Design review of the part built by this model. Coordinates are the model's own, in mm. A direction names the side the tool comes from. Give positions to 0.01 mm unless a question says otherwise; leave off trailing zeros. Write each loop counter-clockwise with the first axis right and the second up, starting at its lowest first coordinate (ties: lowest second). Pieces come first, ordered by that corner, then holes. Notation, with made-up numbers: (9, -20) -> (44, -20) arc R19 cw to (44, -15) -> close; hole circle Ø5 at (40.5, -22.5). An arc over 180 degrees is marked (long way). Answer as a JSON object with one key per item and string values.
```python
from build123d import *

# Parameters (mm, degrees)
F0_R     = 12.5
F1_DEPTH = 20
F2_R     = 50
F3_DEPTH = 40
F4_R     = 34.837403
F5_DEPTH = 100
F7_DEPTH = 25


with BuildPart() as f1:
    # F0 (on Top) → F1 (new body)
    with BuildSketch(Plane.XY):
        with BuildLine():
            ThreePointArc((100, 80), (94.142136, 94.142136), (80, 100))
            Line((80, 100), (-80, 100))
            ThreePointArc((-80, 100), (-94.142136, 94.142136), (-100, 80))
            Line((-100, 80), (-100, -80))
            ThreePointArc((-100, -80), (-94.142136, -94.142136), (-80, -100))
            Line((-80, -100), (80, -100))
            ThreePointArc((80, -100), (94.142136, -94.142136), (100, -80))
            Line((100, -80), (100, 80))
        make_face()
        with Locations((-77, -77)):
            Circle(F0_R, mode=Mode.SUBTRACT)
        with Locations((77, -77)):
            Circle(F0_R, mode=Mode.SUBTRACT)
        with Locations((-77, 77)):
            Circle(F0_R, mode=Mode.SUBTRACT)
        with Locations((77, 77)):
            Circle(F0_R, mode=Mode.SUBTRACT)
    extrude(amount=-F1_DEPTH)

    # F2 (on face) → F3 (join)
    with BuildSketch(Plane.XY):
        Circle(F2_R)
    extrude(amount=F3_DEPTH)

    # F4 (on face) → F5 (cut)
    with BuildSketch(Plane.XY.offset(40)):
        Circle(F4_R)
    extrude(amount=-F5_DEPTH, mode=Mode.SUBTRACT)

    # F6 (on Top) → F7 (cut)
    with BuildSketch(Plane.XY):
        with BuildLine():
            ThreePointArc((-59.309852, -34.015045), (-68.347947, 1.800006), (-57.437243, 37.089687))
            ThreePointArc((-57.437243, 37.089687), (-62.013533, 48.246062), (-74.069896, 48.019696))
            ThreePointArc((-74.069896, 48.019696), (-88.19022, 3.83743), (-77.961014, -41.40436))
            ThreePointArc((-77.961014, -41.40436), (-77.365723, -42.506301), (-76.754857, -43.599686))
            ThreePointArc((-76.754857, -43.599686), (-63.805315, -46.501), (-59.309852, -34.015045))
        make_face()
        with BuildLine():
            ThreePointArc((-77.961014, -41.40436), (-77.426731, -42.53982), (-76.754857, -43.599686))
            ThreePointArc((-76.754857, -43.599686), (-77.365723, -42.506301), (-77.961014, -41.40436))
        make_face()
        with BuildLine():
            ThreePointArc((-54.052199, 69.789687), (-53.014186, 70.58142), (-51.964577, 71.357714))
            ThreePointArc((-51.964577, 71.357714), (-53.059588, 70.641867), (-54.052199, 69.789687))
        make_face()
        with BuildLine():
            ThreePointArc((52.94881, 70.630476), (0.61188, 88.271549), (-51.964577, 71.357714))
            ThreePointArc((-51.964577, 71.357714), (-53.014186, 70.58142), (-54.052199, 69.789687))
            ThreePointArc((-54.052199, 69.789687), (-55.057173, 56.587711), (-42.098027, 53.874279))
            ThreePointArc((-42.098027, 53.874279), (1.351238, 68.358291), (44.194175, 52.168541))
            ThreePointArc((44.194175, 52.168541), (56.583811, 55.06118), (56.54711, 67.783959))
            ThreePointArc((56.54711, 67.783959), (54.766457, 69.230599), (52.94881, 70.630476))
        make_face()
        with BuildLine():
            ThreePointArc((56.54711, 67.783959), (54.909822, 69.411828), (52.94881, 70.630476))
            ThreePointArc((52.94881, 70.630476), (54.766457, 69.230599), (56.54711, 67.783959))
        make_face()
        with BuildLine():
            ThreePointArc((39.419032, -55.864315), (-1.174312, -68.361559), (-41.314479, -54.477479))
            ThreePointArc((-41.314479, -54.477479), (-54.310003, -57.775947), (-52.39069, -71.045453))
            ThreePointArc((-52.39069, -71.045453), (-51.854665, -71.437626), (-51.315704, -71.825756))
            ThreePointArc((-51.315704, -71.825756), (0.860325, -88.269477), (52.705932, -70.811902))
            ThreePointArc((52.705932, -70.811902), (54.044321, -57.453202), (40.883132, -54.801928))
            ThreePointArc((40.883132, -54.801928), (40.154596, -55.337964), (39.419032, -55.864315))
        make_face()
        with BuildLine():
            ThreePointArc((-51.315704, -71.825756), (-51.854665, -71.437626), (-52.39069, -71.045453))
            ThreePointArc((-52.39069, -71.045453), (-51.866142, -71.453438), (-51.315704, -71.825756))
        make_face()
        with BuildLine():
            ThreePointArc((40.883132, -54.801928), (40.12701, -55.299948), (39.419032, -55.864315))
            ThreePointArc((39.419032, -55.864315), (40.154596, -55.337964), (40.883132, -54.801928))
        make_face()
        with BuildLine():
            ThreePointArc((75.178414, -46.264963), (88.273532, -0.155791), (75.341248, 45.999316))
            ThreePointArc((75.341248, 45.999316), (62.161005, 48.55397), (58.316969, 35.690517))
            ThreePointArc((58.316969, 35.690517), (68.371159, 0.257823), (58.58448, -35.249689))
            ThreePointArc((58.58448, -35.249689), (61.853637, -48.331459), (75.178414, -46.264963))
        make_face()
    extrude(amount=-F7_DEPTH, mode=Mode.SUBTRACT)


solid = f1.part
```
(1) For faces 1 (the flat face through (-46, 24, 0)), 2 (the flat face through (100, -1, -10)), 3 (the cylindrical face through (1.398, 88.263, -9.86)), list the 3-axis set-ups (+Z, -Z, +X, -X, +Y, -Y) from which the entire face can be reached by the end or side of a thin tool; tool diameter is ignored.
Here are the results:
{"face 1": "+Z", "face 2": "+Z, -Z, +X, +Y, -Y", "face 3": "+Z, -Z"}
(2) We need section C-C, the plane z = -9.5. Give the number of separate pieces and of enclosed holes in the cut face, then the cut area to 3 significant figures.
Here are the results:
{"separate pieces": "1", "enclosed holes": "9", "area": "25,300 mm²"}
(3) Clearance check with flat-ended pins moving along their axes: pin 1 (1 mm diameter, centred on x = -5.5, z = 11.5, fed in from +Y); pin 2 (1.5 mm diameter, centred on x = 11.5, z = 10, fed in from -Y); pin 3 (1 mm diameter, centred on x = -20.5, z = 18, fed in from -Y). State where each tip first meets the part, or that it passes through.
Here are the results:
{"pin 1": "stops at y = 49.75", "pin 2": "stops at y = -48.83", "pin 3": "stops at y = -45.83"}
(4) We need section A-A, the plane y = 0. State the section outline as (x, z) points, then the cut area to 3 significant figures.
Here are the results:
{"outline": "(-100, -20) -> (-88.27, -20) -> (-88.27, 0) -> (-100, 0) -> close; (-68.37, -20) -> (-34.84, -20) -> (-34.84, 40) -> (-50, 40) -> (-50, 0) -> (-68.37, 0) -> close; (34.84, -20) -> (68.37, -20) -> (68.37, 0) -> (50, 0) -> (50, 40) -> (34.84, 40) -> close; (88.27, -20) -> (100, -20) -> (100, 0) -> (88.27, 0) -> close", "area": "3,020 mm²"}
(5) The part is to be moulded in two halves that separate along X. For faces 4 (the flat face through (-46, 1, -20)), 5 (the cylindrical face through (-54.194, -57.606, -9.86)), 6 (the cylindrical face through (94.297, 93.986, -9.86)), 7 (the cylindrical face through (54.165, -57.62, -9.86)), say which applies: +X half, -X half, draft (parallel to the pull), parting line (faces both ways), or undercut.
Here are the results:
{"face 4": "draft", "face 5": "undercut", "face 6": "+X half", "face 7": "undercut"}
(6) We need section D-D, the plane x = -44.5. State the section outline as (y, z) points, then the cut area to 3 significant figures.
Here are the results:
{"outline": "(-100, -20) -> (-76.24, -20) -> (-76.24, 0) -> (-100, 0) -> close; (-53.43, -20) -> (52.9, -20) -> (52.9, 0) -> (22.8, 0) -> (22.8, 40) -> (-22.8, 40) -> (-22.8, 0) -> (-53.43, 0) -> close; (76.24, -20) -> (100, -20) -> (100, 0) -> (76.24, 0) -> close", "area": "4,900 mm²"}
(7) For line 1 along Y through (x, z) = (-72, -2); line 2 along Y through (x, z) = (-77, -7); line 3 along X through (y, z) = (-25, -12.5), list the stretches that pass through material, from the lowest coordinate up.
Here are the results:
{"line 1": "y = -100 to -88.46, -65.54 to -47.16, 49.17 to 65.54, 88.46 to 100", "line 2": "y = -100 to -89.5, -64.5 to -43.25, 43.17 to 64.5, 89.5 to 100", "line 3": "x = -100 to -84.66, -63.64 to -24.26, 24.26 to 63.64, 84.66 to 100"}
